Design review of the part built by this model. Coordinates are the model's own, in mm. A direction names the side the tool comes from. Round coordinates to 2 decimals unless told otherwise and drop trailing zeros. Order: outer loops, then holes, each group sorted by start corner. A loop starts at its lowest first (then second) coordinate and runs counter-clockwise, first axis right, second up. Notation, with made-up numbers: (-16, 76) - (37, 76) arc R21 ccw to (37, 108) - close; hole circle Ø5 at (19, -7). An arc over 180 degrees is marked (long way). Write item = value, one per line.
Autodesk Inventor part; units mm, degrees
ref_plane "YZ Plane" through (0, 0, 0) normal (1, 0, 0) x (0, 1, 0)
ref_plane "XZ Plane" through (0, 0, 0) normal (0, 1, 0) x (-1, 0, 0)
ref_plane "XY Plane" through (0, 0, 0) normal (0, 0, 1) x (1, 0, 0)
sketch "Sketch1" plane through (0, 0, 0) normal (0, 1, 0) x (-1, 0, 0)
  line L0 (40, 22.5) -> (-40, 22.5)
  line L1 (-40, 22.5) -> (-40, -22.5)
  line L2 (-40, -22.5) -> (40, -22.5)
  line L3 (40, -22.5) -> (40, 22.5)
  line L4 (40, 22.5) -> (-40, -22.5) construction
  line L5 (-40, 22.5) -> (40, -22.5) construction
  point P0 (0, 0)
  dimension "d0" = 80
  dimension "d1" = 45
extrude "ExtrusionForTopOfCase" add sketch "Sketch1" against normal blind 2.54
sketch "Sketch2" plane through (0, -2.54, 0) normal (0, -1, 0) x (1, 0, 0)
  line L0 (40, 22.5) -> (-40, 22.5)
  line L1 (-40, 22.5) -> (-40, -22.5)
  line L2 (40, 22.5) -> (-40, 22.5)
  line L3 (-40, 22.5) -> (-40, -22.5)
  line L4 (-40, -22.5) -> (40, -22.5)
  line L5 (40, -22.5) -> (40, 22.5)
  line L6 (38.095, 20.595) -> (-38.095, 20.595)
  line L7 (-38.095, 20.595) -> (-38.095, -20.595)
  line L8 (-38.095, -20.595) -> (38.095, -20.595)
  line L9 (38.095, -20.595) -> (38.095, 20.595)
  line L10 (38.095, 20.595) -> (-38.095, -20.595) construction
  line L11 (-38.095, 20.595) -> (38.095, -20.595) construction
  point P0 (0, 0)
  dimension "d6" = 1.905
  dimension "d7" = 1.905
extrude "ExtrusionForBottomRidge" add sketch "Sketch2" along normal blind 2.54 contours L9 L8 L7 L6
sketch "Sketch8" plane through (0, 0, 0) normal (0, 1, 0) x (1, 0, 0)
  line L0 (-34.92, -17.42) -> (34.92, -17.42) construction
  line L1 (34.92, -17.42) -> (34.92, 17.42) construction
  line L2 (34.92, 17.42) -> (-34.92, 17.42) construction
  line L3 (-34.92, 17.42) -> (-34.92, -17.42) construction
  line L4 (38.095, 20.595) -> (-38.095, 20.595) construction
  line L5 (-38.095, 20.595) -> (-38.095, -20.595) construction
  line L6 (-38.095, -20.595) -> (38.095, -20.595) construction
  line L7 (38.095, -20.595) -> (38.095, 20.595) construction
  point P0 (0, 0)
  dimension "d39" = 3.175
  dimension "d40" = 3.175
  dimension "d41" = 3.175
  dimension "d42" = 3.175
sketch "Sketch11" plane through (0, 0, 0) normal (0, 1, 0) x (1, 0, 0)
  line L0 (40, -22.5) -> (-40, -22.5)
  line L1 (-40, 22.5) -> (40, 22.5)
  line L2 (-19.426, -22.5) -> (19.436, -22.5)
  line L3 (19.436, -22.5) -> (19.436, 22.5)
  line L4 (19.436, 22.5) -> (-19.426, 22.5)
  line L5 (-19.426, 22.5) -> (-19.426, -22.5)
  line L6 (-40, 22.5) -> (-40, -22.5)
  line L7 (-38.095, -20.595) -> (38.095, -20.595)
  line L8 (-38.095, 20.595) -> (38.095, 20.595)
  line L9 (-18.156, -20.595) -> (18.166, -20.595)
  line L10 (18.166, -20.595) -> (18.166, 20.595)
  line L11 (18.166, 20.595) -> (-18.156, 20.595)
  line L12 (-18.156, 20.595) -> (-18.156, -20.595)
  point P0 (0, 0)
  dimension "d57" = 20.574
  dimension "d58" = 1.27
  dimension "d59" = 1.27
  dimension "d60" = 59.436
extrude "Extrusion7" add sketch "Sketch11" along normal blind 6 contours L0 L5 L7 L3 | L7 L10 L8 L3 | L5 L8 L12 L7 | L8 L5 L1 L3
sketch "Sketch13" plane through (-19.426, 0, -22.5) normal (-1, 0, 0) x (0, 0, 1)
  line L0 (43.095, 6) -> (1.905, 6) construction
  line L1 (22.5, 6) -> (22.5, 0) construction
  line L2 (12.5, 0.5) -> (32.5, 0.5)
  line L3 (32.5, 0.5) -> (32.5, 5.5)
  line L4 (32.5, 5.5) -> (12.5, 5.5)
  line L5 (12.5, 5.5) -> (12.5, 0.5)
  line L6 (12.5, 0.5) -> (32.5, 5.5) construction
  line L7 (32.5, 0.5) -> (12.5, 5.5) construction
  line L8 (0, 6) -> (45, 6)
  point P0 (22.5, 3)
  dimension "d70" = 5
  dimension "d71" = 20
extrude "Extrusion8" cut sketch "Sketch13" against normal up to next
fillet "Fillet1" radius 0.4233 8 edges at (-18.156, 0.5, 0) (-18.156, 3, 10) (-18.156, 5.5, 0) (-18.156, 3, -10) (-19.426, 0.5, 0) (-19.426, 5.5, 0) (-19.426, 3, 10) (-19.426, 3, -10)
hole "Hole7" at (-34.92, 0, -17.42) at (34.92, 0, -17.42) at (34.92, 0, 17.42) at (-34.92, 0, 17.42) direction (0, -1, 0) diameter 3.81 end through all
sketch "Sketch21" plane through (0, -5.08, 0) normal (0, -1, 0) x (1, 0, 0)
  circle A0 centre (34.92, 17.42) radius 1.905
  circle A1 centre (-34.92, -17.42) radius 1.905
  circle A2 centre (34.92, -17.42) radius 1.905
  circle A3 centre (-34.92, 17.42) radius 1.905
  line L0 (38.095, 20.595) -> (-38.095, 20.595)
  line L1 (-38.095, 20.595) -> (-38.095, -20.595)
  line L2 (-38.095, -20.595) -> (38.095, -20.595)
  line L3 (38.095, -20.595) -> (38.095, 20.595)
  circle A4 centre (-14.346, 17.42) radius 1.2657
  circle A5 centre (14.356, 17.42) radius 1.2657
  circle A6 centre (14.356, -17.42) radius 1.2657
  circle A7 centre (-14.346, -17.42) radius 1.2657
  point P0 (0, 0)
hole "Hole12" at (-14.346, -5.08, 17.42) at (14.356, -5.08, 17.42) at (14.356, -5.08, -17.42) at (-14.346, -5.08, -17.42) direction (0, 1, 0) diameter 3.8354 end through all counterbore diameter 4.8514 counterbore depth 3.81
sketch "Sketch22" plane through (0, 0, 0) normal (0, 1, 0) x (1, 0, 0)
  line L0 (40, -22.5) -> (40, 22.5)
  line L1 (19.436, -22.5) -> (40, -22.5)
  circle A0 centre (12.48, 10.5) radius 3.175
  circle A1 centre (12.48, -10.5) radius 3.175
  circle A2 centre (-0.1, -10.5) radius 3.175
  circle A3 centre (-0.1, 10.5) radius 3.175
  point P0 (0, 0)
  dimension "d130" = 27.52
  dimension "d131" = 12
  dimension "d132" = 12.58
  dimension "d133" = 21
  dimension "d134" = 12.58
  dimension "d135" = 21
  dimension "d136" = 6.35
extrude "Extrusion10" add sketch "Sketch22" along normal blind 3.1
sketch "Sketch24" plane through (0, -5.08, 0) normal (0, -1, 0) x (1, 0, 0)
  circle A0 centre (-0.1, -10.5) radius 3.175
  circle A1 centre (12.48, -10.5) radius 3.175
  circle A2 centre (12.48, 10.5) radius 3.175
  circle A3 centre (-0.1, 10.5) radius 3.175
  circle A4 centre (-0.1, -10.5) radius 3.175
  point P0 (0, 0)
hole "Hole14" at (-0.1, -5.08, -10.5) at (-0.1, -5.08, 10.5) at (12.48, -5.08, 10.5) at (12.48, -5.08, -10.5) direction (0, 1, 0) diameter 2.4384 end through all counterbore diameter 3.2639 counterbore depth 3.9878
equation "\"d0\" = CaseLength"
equation "\"d1\" = CaseWidth"
equation "\"d2\" = TopExtensionHeight"
equation "\"d8\" = LowerExtenstionHeight"
equation "\"d58\" = CaseWallThickness"
equation "\"d59\" = CaseWallThickness"
equation "\"d70\" = PiRibbonCableThickness"
equation "\"d71\" = PiRibbonCableWidth"
equation "\"d74\" = FilletForRibbonCable"
equation "\"TopTotalHeight\" = 5.08"
equation "\"TopExtensionHeight\" = 0.5 * TopTotalHeight"
equation "\"LowerExtenstionHeight\" = 0.5 * TopTotalHeight"
properties part number "CaseTopForPiZeroWandCamera" material "Polypropylene"
1) We need section B-B on y = 1.75. Give the number of separate pieces and of enclosed holes in the cut face, and give its area (3 significant figures).
Findings:
separate_pieces = 5
enclosed_holes = 4
area = 335 mm^2
2) We need section A-A on x = -34.92. Write out the cut boundary in (y, z) (3 decimals).
Findings:
outline = (-5.08, -20.595) - (-2.54, -20.595) - (-2.54, -22.5) - (0, -22.5) - (0, -19.325) - (-5.08, -19.325) - close; (-5.08, -15.515) - (0, -15.515) - (0, 15.515) - (-5.08, 15.515) - close; (-5.08, 19.325) - (0, 19.325) - (0, 22.5) - (-2.54, 22.5) - (-2.54, 20.595) - (-5.08, 20.595) - close
3) We need section C-C on z = 2.5. Write out the cut boundary in (x, y) (3 decimals).
Findings:
outline = (-40, -2.54) - (-38.095, -2.54) - (-38.095, -5.08) - (38.095, -5.08) - (38.095, -2.54) - (40, -2.54) - (40, 0) - (19.436, 0) - (19.436, 6) - (18.166, 6) - (18.166, 0) - (-18.156, 0) - (-18.156, 0.077) arc R0.423 ccw to (-18.579, 0.5) - (-19.003, 0.5) arc R0.423 ccw to (-19.426, 0.077) - (-19.426, 0) - (-40, 0) - close; (-19.426, 5.923) arc R0.423 ccw to (-19.003, 5.5) - (-18.579, 5.5) arc R0.423 ccw to (-18.156, 5.923) - (-18.156, 6) - (-19.426, 6) - close
4) The part is to be moulded in two halves that separate along Z. For faces 4 (the flat face through (-1, 1, 22.5)), 5 (the cylindrical face through (-15.642, -0.626, -16.007)), 6 (the flat face through (40, -1, 0)), say which applies: released by +Z, released by -Z, zero draft, split by the parting line, or undercut.
Findings:
face_4 = released by +Z
face_5 = undercut
face_6 = zero draft
5) For faces 1 (the flat face through (-1, -4, -20.595)), 2 (the flat face through (14, 3.1, -11)), 3 (the cylindrical face through (-15.075, -3.148, 15.106)), list the 3-axis set-ups (+Z, -Z, +X, -X, +Y, -Y) from which the entire face can be reached by the end or side of a thin tool; tool diameter is ignored.
Findings:
face_1 = -Z, +X, -X, -Y
face_2 = +Y
face_3 = -Y
6) Clearance check with flat-ended pins moving along their axes: pin 1 Ø2 at (y, z) = (-4, 0.5) entering from +X (3 decimals); pin 2 Ø5 at (y, z) = (-3.5, -17.5) entering from +X; pin 3 Ø3 at (y, z) = (4.5, -7.5) entering from -X; pin 4 Ø5 at (x, z) = (-14.346, -17.42) entering from +Y. State where each tip first meets the part, or that it passes through.
Findings:
pin_1 = 38.095
pin_2 = 40
pin_3 = -19.43
pin_4 = 0
7) To check wall thickness, follow L1, parallel to X at y = -2.7, z = 17.42 (3 decimals); L2, parallel to X at y = -2.15, z = 17.42 (3 decimals); L3, parallel to Z at x = 35, y = -0.75. State the ranges of each line that lie inside material, in increasing order. Write a range as from..to.
Findings:
L1 = -38.095..-36.825, -33.015..-16.772, -11.92..11.93, 16.782..33.015, 36.825..38.095
L2 = -40..-36.825, -33.015..-16.772, -11.92..11.93, 16.782..33.015, 36.825..40
L3 = -22.5..-19.32, -15.52..15.52, 19.32..22.5
8) We need section D-D on x = -7.5. Write out the cut boundary in (y, z) (3 decimals), and give its area (3 significant figures).
Findings:
outline = (-5.08, -20.595) - (-2.54, -20.595) - (-2.54, -22.5) - (6, -22.5) - (6, -20.595) - (0, -20.595) - (0, 20.595) - (6, 20.595) - (6, 22.5) - (-2.54, 22.5) - (-2.54, 20.595) - (-5.08, 20.595) - close
area = 242 mm^2
